Autodesk Inventor part; units mm, degrees
ref_plane "YZ Plane" through (0, 0, 0) normal (1, 0, 0) x (0, 1, 0)
ref_plane "XZ Plane" through (0, 0, 0) normal (0, 1, 0) x (-1, 0, 0)
ref_plane "XY Plane" through (0, 0, 0) normal (0, 0, 1) x (1, 0, 0)
sketch "Sketch1" plane through (0, 0, 0) normal (0, 0, 1) x (1, 0, 0)
  circle A0 centre (0, 0) radius 11.25
  arc A1 (-32.7929, -17.201) -> (-31.2929, -19.799) centre (0, 0) ccw
  line L0 (-32.7929, -17.201) -> (-31.0547, -16.1974)
  line L1 (-32.7929, -17.201) -> (-31.0547, -16.1974)
  line L2 (-29.5547, -18.7955) -> (-31.2929, -19.799)
  line L3 (-31.2929, -19.799) -> (-29.5547, -18.7955)
  line L4 (-16.1974, -31.0547) -> (-17.201, -32.7929)
  line L5 (-17.201, -32.7929) -> (-16.1974, -31.0547)
  arc A2 (-19.799, -31.2929) -> (-17.201, -32.7929) centre (0, 0) ccw
  line L6 (-19.799, -31.2929) -> (-18.7955, -29.5547)
  line L7 (-19.799, -31.2929) -> (-18.7955, -29.5547)
  arc A3 (17.201, -32.7929) -> (19.799, -31.2929) centre (0, 0) ccw
  line L8 (17.201, -32.7929) -> (16.1974, -31.0547)
  line L9 (17.201, -32.7929) -> (16.1974, -31.0547)
  line L10 (18.7955, -29.5547) -> (19.799, -31.2929)
  line L11 (19.799, -31.2929) -> (18.7955, -29.5547)
  arc A4 (31.2929, -19.799) -> (32.7929, -17.201) centre (0, 0) ccw
  line L12 (31.2929, -19.799) -> (29.5547, -18.7955)
  line L13 (31.0547, -16.1974) -> (32.7929, -17.201)
  line L14 (32.7929, -17.201) -> (31.0547, -16.1974)
  line L15 (32.7929, 17.201) -> (31.0547, 16.1974)
  line L16 (32.7929, 17.201) -> (31.0547, 16.1974)
  arc A5 (32.7929, 17.201) -> (31.2929, 19.799) centre (0, 0) ccw
  line L17 (29.5547, 18.7955) -> (31.2929, 19.799)
  line L18 (31.2929, 19.799) -> (29.5547, 18.7955)
  line L19 (16.1974, 31.0547) -> (17.201, 32.7929)
  line L20 (17.201, 32.7929) -> (16.1974, 31.0547)
  line L21 (19.799, 31.2929) -> (18.7955, 29.5547)
  line L22 (19.799, 31.2929) -> (18.7955, 29.5547)
  line L23 (-17.201, 32.7929) -> (-16.1974, 31.0547)
  line L24 (-17.201, 32.7929) -> (-16.1974, 31.0547)
  line L25 (-18.7955, 29.5547) -> (-19.799, 31.2929)
  line L26 (-19.799, 31.2929) -> (-18.7955, 29.5547)
  arc A6 (-31.2615, 19.7809) -> (-32.7929, 17.201) centre (-0.5443, -0.1969) ccw
  line L27 (-31.2615, 19.7809) -> (-29.5547, 18.7955)
  line L28 (-31.2615, 19.7809) -> (-29.5547, 18.7955)
  line L29 (-31.0547, 16.1974) -> (-32.7929, 17.201)
  line L30 (-32.7929, 17.201) -> (-31.0547, 16.1974)
  arc A7 (-27.9532, 21.6091) -> (-22.3503, 27.212) centre (-22.995, 22.2538) ccw
  circle A8 centre (-22.995, 22.2538) radius 5
  circle A9 centre (21.9063, 22.2538) radius 5
  circle A10 centre (21.9063, 22.2538) radius 5
  circle A11 centre (-22.995, 22.2538) radius 4.75
  circle A12 centre (-22.995, -22.6475) radius 4.75
  circle A13 centre (21.9063, -22.6475) radius 4.75
  circle A14 centre (21.9063, 22.2538) radius 4.75
  circle A15 centre (0, 0) radius 34.775
  circle A16 centre (0, 0) radius 36.75
  point P0 (0, 0)
  point P1 (0, 49.75)
  point P2 (26.6556, 22.3333)
  point P3 (21.9111, 27.0038)
  point P4 (-22.0321, 26.9051)
  point P5 (-27.6123, 21.1391)
  point P6 (-27.5325, -21.2429)
  point P7 (-21.6596, -27.2059)
  point P8 (21.4454, -27.3751)
  point P9 (26.6466, -22.3441)
  dimension "d6" = 70.05
  dimension "d8" = 74.0608
  dimension "d0" = 10
  dimension "d1" = 0.25
  dimension "d4" = 360
  dimension "d7" = 0.25
  dimension "d9" = 73.5
extrude "Extrusion1" add sketch "Sketch1" along normal blind 21.9 contours A0 | A16 A12 | A12 A15 A16 | A15 A7 A9 A13 A12 | A12 A15 | A15 A11 A7 | A11 A15 | A15 A11 | A15 A13 | A13 A15 | A15 A14 A9 | A15 A14 | A14 A15 picked at (20.2713, 26.7736)
sketch "Skizze4" plane through (0, 0, 21.9) normal (0, 0, 1) x (1, 0, 0)
  circle A0 centre (0, 0) radius 11
  dimension "d24" = 22
extrude "Extrusion4" cut sketch "Skizze4" against normal up to surface (21.9 mm away) from surface at 0
sketch "Skizze5" plane through (0, 0, 21.9) normal (0, 0, 1) x (1, 0, 0)
  circle A0 centre (0, 0) radius 11
  circle A1 centre (0, 0) radius 14.17
  dimension "d27" = 28.34
extrude "Extrusion5" cut sketch "Skizze5" against normal blind 8.76 contours A0 | A1
sketch "Skizze6" plane through (0, 0, 0) normal (0, 0, -1) x (-1, 0, 0)
  line L0 (0, 0) -> (-16.92, 0)
  line L1 (-16.92, 0) -> (-16.92, 28.34)
  line L2 (-16.92, 28.34) -> (0, 28.34)
  line L3 (0, 28.34) -> (0, 0)
  circle A0 centre (-16.92, 28.34) radius 1.7
  circle A1 centre (16.92, 28.34) radius 1.7
  dimension "d30" = 16.92
  dimension "d31" = 28.34
  dimension "d32" = 3.4
extrude "Extrusion6" cut sketch "Skizze6" against normal through all contours A0 L2 L1 | L1 L2 A0 | A1
sketch "Skizze8" plane through (0, 0, 0) normal (0, 0, -1) x (-1, 0, 0)
  circle A0 centre (-16.92, 28.34) radius 1.7
  circle A1 centre (-16.92, 28.34) radius 2.855
  circle A2 centre (16.92, 28.34) radius 1.7
  circle A3 centre (16.92, 28.34) radius 2.855
  point P0 (0, 0)
  dimension "d39" = 5.71
  dimension "d40" = 5.71
extrude "Extrusion8" cut sketch "Skizze8" against normal blind 3.29 contours A1 | A2 | A3
properties part number "2024_08_22_LED_blende"
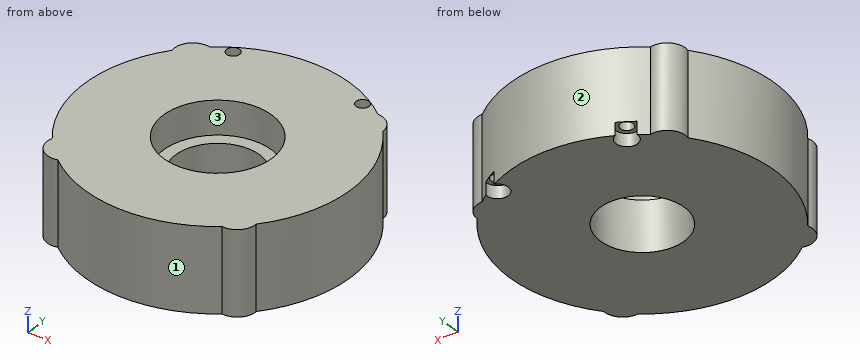
Read the model definition and answer for the solid it produces. Units are mm, in the model's axes. Face numbers are marked on the shaded views. Round coordinates to 2 decimals unless told otherwise and drop trailing zeros. Loops run counter-clockwise (first coordinate to the right, second up) from the corner with the lowest first, then second, coordinate; pieces in that order, holes last.
Q1. Section A-A on x = 0 is taken. Write down the section's boundary in (y, z) (3 decimals), and give its area (3 significant figures).
Q2. Section D-D on x = 13 is taken. Write down the section's boundary in (y, z), and give its area (3 significant figures).
Q3. Consider probe 1 along Y at (x, z) = (0, 17.25) (3 decimals); probe 2 along Y at (x, z) = (0, 5) (3 decimals); probe 3 along X at (y, z) = (28.34, 0.85) (3 decimals). Determine where each line is inside the solid, lowest interval first.
Q4. Determine the mould class of the marked faces 1, 2 and 3 for opening direction Y: released by +Y, released by -Y, zero draft, split by the parting line, or undercut.
Q5. Section C-C on z = 18 is taken. Give the number of separate pieces and of enclosed holes in the cut face, and give its area (3 significant figures).
Q6. Each of these flat-tipped pins is pushed along its axis until it touches: pin 1 (22.5 mm diameter, centred on x = 0, y = 0, fed in from +Z); pin 2 (1 mm diameter, centred on y = -8, z = 18.5, fed in from -X); pin 3 (2 mm diameter, centred on x = -2.5, z = 2.5, fed in from +Y); pin 4 (13 mm diameter, centred on x = 0, y = 0, fed in from -Z). Where does it stop, or does it pass through?
Output:
1. outline: (-34.775, 0) - (-11, 0) - (-11, 13.14) - (-14.17, 13.14) - (-14.17, 21.9) - (-34.775, 21.9) - close; (11, 0) - (34.775, 0) - (34.775, 21.9) - (14.17, 21.9) - (14.17, 13.14) - (11, 13.14) - close
1. area: 986 mm2
2. outline: (-32.25, 0) - (32.25, 0) - (32.25, 21.9) - (5.64, 21.9) - (5.64, 13.14) - (-5.64, 13.14) - (-5.64, 21.9) - (-32.25, 21.9) - close
2. area: 1,310 mm2
3. probe 1: y = -34.775 to -14.17, 14.17 to 34.775
3. probe 2: y = -34.775 to -11, 11 to 34.775
3. probe 3: x = -20.153 to -19.775, -14.065 to 14.065, 19.775 to 20.153
4. face 1: released by -Y
4. face 2: released by +Y
4. face 3: undercut
5. separate pieces: 1
5. enclosed holes: 3
5. area: 3,190 mm2
6. pin 1: stops at z = 13.14
6. pin 2: stops at x = -33.96
6. pin 3: stops at y = 34.74
6. pin 4: passes through
